from build123d import *

# Parameters (mm, degrees)
SKETCH2_W           = 16
SKETCH2_H           = 16
BOSS_EXTRUDE1_DEPTH = 11
SKETCH3_R           = 1.5
BOSS_EXTRUDE2_DEPTH = 3
SKETCH4_W           = 16
SKETCH4_H           = 16
SKETCH4_W_2         = 13
SKETCH4_H_2         = 13
CUT_EXTRUDE1_DEPTH  = 5
BOSS_EXTRUDE3_DEPTH = 3.5
SKETCH6_W           = 16
SKETCH6_H           = 16
SKETCH6_W_2         = 11
SKETCH6_H_2         = 11
CUT_EXTRUDE2_DEPTH  = 5.5
BOSS_EXTRUDE4_DEPTH = 0.5
BOSS_EXTRUDE5_START = -0.5
BOSS_EXTRUDE5_DEPTH = 0.5
BOSS_EXTRUDE6_DEPTH = 11
SKETCH10_R          = 1
BOSS_EXTRUDE7_DEPTH = 3.5


with BuildPart() as part:
    # Sketch2 → Boss-Extrude1 (new body)
    with BuildSketch(Plane(origin=(0, 0, 0), x_dir=(1, 0, 0), z_dir=(0, 1, 0))):
        with Locations((8, 8)):
            Rectangle(SKETCH2_W, SKETCH2_H)
    extrude(amount=BOSS_EXTRUDE1_DEPTH)

    # Sketch3 → Boss-Extrude2 (add)
    with BuildSketch(Plane.XZ):
        with Locations(Location((8, -8, 0), (0, 0, 270))):
            Circle(SKETCH3_R)
    extrude(amount=BOSS_EXTRUDE2_DEPTH)

    # Sketch4 → Cut-Extrude1 (cut)
    with BuildSketch(Plane.XZ):
        with Locations((8, -8)):
            Rectangle(SKETCH4_W, SKETCH4_H)
        with Locations((8, -8)):
            Rectangle(SKETCH4_W_2, SKETCH4_H_2, mode=Mode.SUBTRACT)
    extrude(amount=-CUT_EXTRUDE1_DEPTH, mode=Mode.SUBTRACT)

    # Sketch5 → Boss-Extrude3 (add)
    with BuildSketch(Plane(origin=(0, 11, 0), x_dir=(1, 0, 0), z_dir=(0, 1, 0))):
        Polygon((7.5, 10), (7.5, 8.5), (6, 8.5), (6, 7.5), (7.5, 7.5), (7.5, 6), (8.5, 6), (8.5, 7.5), (10, 7.5), (10, 8.5), (8.5, 8.5), (8.5, 10), align=None)
    extrude(amount=BOSS_EXTRUDE3_DEPTH)

    # Sketch6 → Cut-Extrude2 (cut)
    with BuildSketch(Plane(origin=(0, 11, 0), x_dir=(1, 0, 0), z_dir=(0, 1, 0))):
        with Locations((8, 8)):
            Rectangle(SKETCH6_W, SKETCH6_H)
        with Locations((8, 8)):
            Rectangle(SKETCH6_W_2, SKETCH6_H_2, mode=Mode.SUBTRACT)
    extrude(amount=-CUT_EXTRUDE2_DEPTH, mode=Mode.SUBTRACT)

    # Sketch7 → Boss-Extrude4 (add)
    with BuildSketch(Plane.ZY.offset(-2.5)):
        with BuildLine():
            Line((-13.5, 11), (-13.582711823, 11))
            ThreePointArc((-13.582711823, 11), (-13.903085543, 10.883875865), (-14.074646778, 10.589442719))
            Line((-14.074646778, 10.589442719), (-15, 5.5))
            Line((-15, 5.5), (-13.5, 5.5))
            Line((-13.5, 5.5), (-13.5, 11))
        make_face()
    extrude(amount=-BOSS_EXTRUDE4_DEPTH)

    # Sketch8 → Boss-Extrude5 (add)
    with BuildSketch(Plane(origin=(13.5, 0, 0), x_dir=(0, 0, -1), z_dir=(1, 0, 0)).offset(BOSS_EXTRUDE5_START)):
        with BuildLine():
            Line((15, 5.5), (13.5, 5.5))
            Line((13.5, 5.5), (13.5, 11))
            Line((13.5, 11), (13.582711823, 11))
            ThreePointArc((13.582711823, 11), (13.903085543, 10.883875865), (14.074646778, 10.589442719))
            Line((14.074646778, 10.589442719), (15, 5.5))
        make_face()
    extrude(amount=BOSS_EXTRUDE5_DEPTH)

    # Sketch9 → Boss-Extrude6 (add)
    with BuildSketch(Plane.ZY.offset(-2.5)):
        with BuildLine():
            Line((-2.5, 11), (-2.417288177, 11))
            ThreePointArc((-2.417288177, 11), (-2.096914457, 10.883875865), (-1.925353222, 10.589442719))
            Line((-1.925353222, 10.589442719), (-1, 5.5))
            Line((-1, 5.5), (-2.5, 5.5))
            Line((-2.5, 5.5), (-2.5, 11))
        make_face()
    extrude(amount=-BOSS_EXTRUDE6_DEPTH)

    # Sketch10 → Boss-Extrude7 (add)
    with BuildSketch(Plane.XZ):
        with Locations(Location((4.3, -10.65, 0), (0, 0, 270))):
            Circle(SKETCH10_R)
        with Locations(Location((10.55, -13.15, 0), (0, 0, 270))):
            Circle(SKETCH10_R)
    extrude(amount=BOSS_EXTRUDE7_DEPTH)


solid = part.part
Can you work these out from the model? Positions are in its coordinate system, mm. A direction names the side the tool comes from. Coordinates: 2 decimals unless noted, no trailing zeros. Loops run counter-clockwise (first coordinate to the right, second up) from the corner with the lowest first, then second, coordinate; pieces in that order, holes last. Notation, with made-up numbers: M 49.25,29.5 L 82.25,29.5 A32 cw 82.25,59.5 Z; hole C 34,-36.75 d5. An arc over 180 degrees is marked long. Answer as CSV lines item,"result". Start each with the question number.
1. Suppose I cut it at B-B, the plane x = 2.75. List the corners of the cut face in (y, z) for me, plus the area to 3 significant figures.
2. Suppose I cut it at D-D, the plane z = -8. List the corners of the cut face in (x, y) for me, plus the area to 4 significant figures.
3. If I drill on probe 1 along X at (y, z) = (11.5, -6.75); probe 2 along Y at (x, z) = (8.25, -6.25); probe 3 along Z at (x, y) = (9, 2.25), over which ranges is the centre line in solid material (lowest first)? Write a range as [from, to].
4. For pin 1 Ø2.5 at (x, y) = (6.5, 3) entering from -Z; pin 2 Ø1.6 at (y, z) = (8, -11.5) entering from +X; pin 3 Ø0.8 at (x, y) = (8, 12) entering from +Z, each with a flat end and sliding along its axis, tell me the tip position at first contact or that it passes through.
5. Thinking about a two-plate mould opening in X: for faces 6 (the face through (13, 8, -14)), 7 (the face through (8, -3, -8)), 8 (the face through (8.5, 13, -9)), 9 (the face through (8, 8, -13.5)), which applies, +X half, -X half, draft (parallel to the pull), parting line (faces both ways), or undercut?
6. Suppose I cut it at C-C, the plane y = 13.25. List the corners of the cut face in (x, z) for me.
7. For faces 1 (the face through (8, 2, -14.5)), 2 (the face through (9.94, -1.73, -12.36)), 3 (the face through (8, 13, -10)), 4 (the face through (2, 5.5, -8)), 5 (the face through (8, 13, -6)), which set-ups out of +Z, -Z, +X, -X, +Y, -Y let a thin tool reach every point of the face, with its end or its side?
8. Suppose I cut it at A-A, the plane z = -13.15. List the corners of the cut face in (x, y) for me.
Output:
1,outline,"M 0,-14.5 L 5,-14.5 L 5,-16 L 5.5,-16 L 5.5,-15 L 10.59,-14.07 A0.5 ccw 11,-13.58 L 11,-2.42 A0.5 ccw 10.59,-1.93 L 5.5,-1 L 5.5,0 L 5,0 L 5,-1.5 L 0,-1.5 Z"
1,area,"144 mm^2"
2,outline,"M 0,5 L 1.5,5 L 1.5,0 L 6.5,0 L 6.5,-3 L 9.5,-3 L 9.5,0 L 14.5,0 L 14.5,5 L 16,5 L 16,5.5 L 13.5,5.5 L 13.5,11 L 10,11 L 10,14.5 L 6,14.5 L 6,11 L 2.5,11 L 2.5,5.5 L 0,5.5 Z"
2,area,"156.5 mm^2"
3,probe 1,"x = [7.5, 8.5]"
3,probe 2,"y = [0, 14.5]"
3,probe 3,"z = [-14.5, -1.5]"
4,pin 1,"stops at z = -14.5"
4,pin 2,"stops at x = 13.5"
4,pin 3,"stops at z = -6"
5,face 6,"undercut"
5,face 7,"draft"
5,face 8,"+X half"
5,face 9,"undercut"
6,outline,"M 6,-8.5 L 7.5,-8.5 L 7.5,-10 L 8.5,-10 L 8.5,-8.5 L 10,-8.5 L 10,-7.5 L 8.5,-7.5 L 8.5,-6 L 7.5,-6 L 7.5,-7.5 L 6,-7.5 Z"
7,face 1,"-Z, +X, -X, -Y"
7,face 2,"-Y"
7,face 3,"-Z, +X, -X, +Y"
7,face 4,"+Y"
7,face 5,"+Z, +X, -X, +Y"
8,outline,"M 0,5 L 1.5,5 L 1.5,0 L 9.55,0 L 9.55,-3.5 L 11.55,-3.5 L 11.55,0 L 14.5,0 L 14.5,5 L 16,5 L 16,5.5 L 13.5,5.5 L 13.5,11 L 2.5,11 L 2.5,5.5 L 0,5.5 Z"
